Verification items for the finished model (mm, model axes). A direction names the side the tool comes from. Give positions to 0.01 mm unless a question says otherwise; leave off trailing zeros. Loops run counter-clockwise (first coordinate to the right, second up) from the corner with the lowest first, then second, coordinate; pieces in that order, holes last. Notation, with made-up numbers: M 2,-9 L 19,-9 A21 ccw 19,17 Z; hole C -35,20 d6. An arc over 180 degrees is marked long. Answer in a Markdown table with one row per item.
Autodesk Fusion 360 part; units mm, degrees
sketch "doorStop" plane through (0, 0, 0) normal (0, 0, 1) x (1, 0, 0)
  circle A0 centre (0, 0) radius 18.5
  circle A1 centre (0, 0) radius 14.5
  line L0 (0, 0) -> (-12.325, 0) construction
  line L1 (-12.325, 0) -> (-14.5, 0)
  line L2 (-14.5, 0) -> (-14.5, 16.5)
  line L3 (-14.5, 16.5) -> (-12.325, 16.5)
  line L4 (-12.325, 16.5) -> (-12.325, 0)
  line L5 (-12.325, 0) -> (-14.5, 0)
  line L6 (-14.5, 0) -> (-14.5, -16.5)
  line L7 (-14.5, -16.5) -> (-12.325, -16.5)
  line L8 (-12.325, -16.5) -> (-12.325, 0)
  dimension "d4" = 37
  dimension "d5" = 29
  dimension "d6" = 12.325
  dimension "d7" = 2.175
  dimension "d8" = 16.5
  dimension "d9" = 2.175
  dimension "d10" = 16.5
extrude "Extrude1" add sketch "doorStop" along normal blind 10 contours A0 A1 L4 L8 makes body 1
ref_plane "WorkPlane3" through (18.5, 0, 8.3668) normal (1, 0, 0) x (0, -1, 0)
sketch "link" plane through (18.5, 0, 7.5753) normal (1, 0, 0) x (0, 1, 0)
  line L0 (-13.7965, -7.5753) -> (-7.6383, -7.5753)
  line L1 (-7.6383, 2.4247) -> (-13.7965, 2.4247)
  line L2 (-7.6383, -7.5753) -> (7.6383, -7.5753)
  line L3 (7.6383, 2.4247) -> (-7.6383, 2.4247)
  line L4 (13.7965, -7.5753) -> (7.6383, -7.5753)
  line L5 (13.7965, 2.4247) -> (7.6383, 2.4247)
  line L6 (-13.7965, -7.5753) -> (-18.5, -7.5753)
  line L7 (18.5, -7.5753) -> (13.7965, -7.5753)
  line L8 (-13.7965, 2.4247) -> (-18.5, 2.4247)
  line L9 (18.5, 2.4247) -> (13.7965, 2.4247)
  line L10 (18.5, -7.5753) -> (18.5, 2.4247)
  line L11 (-18.5, -7.5753) -> (-18.5, 2.4247)
  line L12 (-18.5, -7.5753) -> (18.5, -7.5753) construction
  line L13 (-18.5, -7.5753) -> (18.5, -7.5753) construction
  line L14 (0, -7.5753) -> (-5, -7.5753) construction
  line L15 (-5, -7.5753) -> (5, -7.5753)
  line L16 (5, -7.5753) -> (5, 2.4247)
  line L17 (5, 2.4247) -> (-5, 2.4247)
  line L18 (-5, 2.4247) -> (-5, -7.5753)
  point P0 (0, -7.5753)
  dimension "d20" = 5
  dimension "d21" = 10
  dimension "d22" = 10
extrude "Extrude2" add sketch "link" along normal blind 3 separate body contours L2 L3 L15 L16 L17 L18 makes body 2
extrude "Extrude3" add 1 faces at (18.5, -1.6667, 6.6667) along direction (-1, 0, 0) blind 1 on bodies 2 bodies 2 1
ref_plane "WorkPlane4" through (21.5, 0, 5) normal (1, 0, 0) x (0, 0, -1)
sketch "doorHolder1" plane through (21.5, 0, 2.5) normal (1, 0, 0) x (0, 1, 0)
  line L0 (-5, 7.5) -> (-5, -2.5)
  line L1 (-5, -2.5) -> (5, -2.5)
  line L2 (5, -2.5) -> (5, 7.5)
  line L3 (5, 7.5) -> (-5, 7.5)
  line L4 (-5, -2.5) -> (5, -2.5) construction
  line L5 (0, -2.5) -> (-15, -2.5) construction
  line L6 (-15, -2.5) -> (15, -2.5)
  line L7 (15, -2.5) -> (15, 17.5)
  line L8 (15, 17.5) -> (-15, 17.5)
  line L9 (-15, 17.5) -> (-15, -2.5)
  point P0 (0, -2.5)
  dimension "d31" = 15
  dimension "d32" = 30
  dimension "d33" = 20
extrude "Extrude4" add sketch "doorHolder1" along normal blind 5 bodies 2
ref_plane "WorkPlane5" through (26.5, 0, 10) normal (1, 0, 0) x (0, 0, -1)
sketch "doorHolderBottom" plane through (26.5, 0, 10) normal (1, 0, 0) x (0, 1, 0)
  line L0 (-15, 10) -> (-15, -10)
  line L1 (-15, -10) -> (15, -10)
  line L2 (15, -10) -> (15, 10)
  line L3 (15, 10) -> (-15, 10)
  line L4 (-15, -10) -> (15, -10)
  line L5 (15, -10) -> (15, -5)
  line L6 (15, -5) -> (-15, -5)
  line L7 (-15, -5) -> (-15, -10)
  dimension "d37" = 30
  dimension "d38" = 5
extrude "Extrude5" add sketch "doorHolderBottom" along normal blind 39 contours L0 L1 L2 L4 L5 L6 L7 bodies 2
ref_plane "WorkPlane6" through (65.5, 0, 2.5) normal (1, 0, 0) x (0, 0, -1)
sketch "doorHolder2" plane through (65.5, 0, 2.5) normal (1, 0, 0) x (0, 1, 0)
  line L0 (0, -2.5) -> (-15, -2.5) construction
  line L1 (-15, -2.5) -> (15, -2.5)
  line L2 (15, 17.5) -> (-15, 17.5)
  line L3 (15, -2.5) -> (15, 17.5)
  line L4 (-2.5, 2.5) -> (-2.5, -2.5)
  line L5 (-15, 17.5) -> (-15, -2.5)
  line L6 (2.5, 2.5) -> (-2.5, 2.5)
  line L7 (-2.5, -2.5) -> (2.5, -2.5) construction
  line L8 (2.5, -2.5) -> (2.5, 2.5)
  line L9 (-2.5, -2.5) -> (2.5, -2.5)
  point P0 (0, -2.5)
  dimension "d43" = 15
  dimension "d44" = 30
  dimension "d45" = 20
extrude "Extrude6" add sketch "doorHolder2" along normal blind 5 bodies 2
equation "doorStopDiameter = 29 mm"
equation "doorStopHolderThickness = 4 mm"
equation "d4 = doorStopDiameter + ( 2 * doorStopHolderThickness )"
equation "d5 = doorStopDiameter"
equation "d6 = ( doorStopDiameter / 2 ) * ( doorStopHolderClosurePercent )"
equation "d7 = ( doorStopDiameter / 2 ) * ( 1 - doorStopHolderClosurePercent )"
equation "d8 = ( doorStopDiameter + doorStopHolderThickness ) / 2"
equation "d9 = ( doorStopDiameter / 2 ) * ( 1 - doorStopHolderClosurePercent )"
equation "d10 = ( doorStopDiameter + doorStopHolderThickness ) / 2"
equation "d11 = doorStopHeight"
equation "doorStopHeight = 10 mm"
equation "linkLength = 3 mm"
equation "linkThickness = 10 mm"
equation "d20 = linkThickness / 2"
equation "d21 = linkThickness"
equation "d22 = doorStopHeight"
equation "d23 = linkLength"
equation "doorHolderHeight = 15 mm"
equation "doorHolderWidth = 30 mm"
equation "doorHolderThickness = 5 mm"
equation "d31 = doorHolderWidth / 2"
equation "d32 = doorHolderWidth"
equation "d33 = doorHolderHeight + doorHolderThickness"
equation "d34 = doorHolderThickness"
equation "d37 = doorHolderWidth"
equation "d38 = doorHolderThickness"
equation "d39 = doorThickness"
equation "doorThickness = 39 mm"
equation "d43 = doorHolderWidth / 2"
equation "d44 = doorHolderWidth"
equation "d45 = doorHolderHeight + doorHolderThickness"
equation "d46 = doorHolderThickness"
Item 1: Sectioned sample at C-C (y = 0). Record the cut outline in (x, z), and give its area (3 significant figures).
Reported:
| item | result |
|---|---|
| outline | M 14.5,0 L 70.5,0 L 70.5,20 L 65.5,20 L 65.5,5 L 26.5,5 L 26.5,20 L 21.5,20 L 21.5,10 L 14.5,10 Z |
| area | 465 mm^2 |
Item 2: Sectioned sample at B-B (z = 11.5). Record the cut outline in (x, y), and give its area (3 significant figures).
Reported:
| item | result |
|---|---|
| outline | M 21.5,-15 L 26.5,-15 L 26.5,15 L 21.5,15 Z; M 65.5,-15 L 70.5,-15 L 70.5,15 L 65.5,15 Z |
| area | 300 mm^2 |
Item 3: Tool access check on faces 4 (the flat face through (26.5, 0, 13)), 5 (the flat face through (46, 15, 3)), 6 (the flat face through (46, -15, 3)). Record the directions out of +Z, -Z, +X, -X, +Y, -Y that give a thin tool (end or side, any length) a straight path to the whole face; none if there is none.
Reported:
| item | result |
|---|---|
| face 4 | +Z, +Y, -Y |
| face 5 | +Z, -Z, +X, +Y |
| face 6 | +Z, -Z, +X, -Y |
Item 4: Sectioned sample at D-D (y = -10). Record the cut outline in (x, z) (3 decimals).
Reported:
| item | result |
|---|---|
| outline | M -12.325,0 L -10.5,0 L -10.5,10 L -12.325,10 Z; M 10.5,0 L 15.564,0 L 15.564,10 L 10.5,10 Z; M 21.5,0 L 70.5,0 L 70.5,20 L 65.5,20 L 65.5,5 L 26.5,5 L 26.5,20 L 21.5,20 Z |
Item 5: Go/stop test with flat-tipped pins: pin 1 (15 mm diameter, centred on x = 43.5, y = 4, fed in from +Z); pin 2 (1.5 mm diameter, centred on y = -5, z = 17, fed in from -X); pin 3 (17 mm diameter, centred on x = 3.5, y = -5.5, fed in from +Z). Record where each tip stops, or that it passes through.
Reported:
| item | result |
|---|---|
| pin 1 | stops at z = 5 |
| pin 2 | stops at x = 21.5 |
| pin 3 | stops at z = 10 |
Item 6: Scan lines: L1, parallel to X at y = 0, z = 7.25; L2, parallel to Y at x = 0, z = 6; L3, parallel to X at y = 3, z = 18. Record each from-to range of solid material in increasing order. Write a range as [from, to].
Reported:
| item | result |
|---|---|
| L1 | x = [14.5, 26.5], [65.5, 70.5] |
| L2 | y = [-18.5, -14.5], [14.5, 18.5] |
| L3 | x = [21.5, 26.5], [65.5, 70.5] |
Item 7: Sectioned sample at A-A (x = 0). Record the cut outline in (y, z), and give its area (3 significant figures).
Reported:
| item | result |
|---|---|
| outline | M -18.5,0 L -14.5,0 L -14.5,10 L -18.5,10 Z; M 14.5,0 L 18.5,0 L 18.5,10 L 14.5,10 Z |
| area | 80.0 mm^2 |
Item 8: Release check for a two-part mould opening along X. For faces 1 (the flat face through (21.5, 0, 12)), 2 (the flat face through (68, 0, 20)), 3 (the flat face through (-12.325, 11, 5)) record: released by +X, released by -X, zero draft, split by the parting line, or undercut.
Reported:
| item | result |
|---|---|
| face 1 | undercut |
| face 2 | zero draft |
| face 3 | released by -X |
